from build123d import *

# Parameters (mm, degrees)
F1_DEPTH = 5
F2_W     = 20
F2_H     = 20
F3_DEPTH = 5
F6_W     = 10
F6_H     = 10
F6_R     = 3
F9_DEPTH = 10
F10_R    = 2


with BuildPart() as f1:
    # F0 (on Top) → F1 (new body)
    with BuildSketch(Plane.XY):
        with BuildLine():
            Line((-11.8750007629, -7.425), (-12.575, -7.425))
            Line((-12.575, -7.425), (-13.375, -7.425))
            Line((-13.375, -7.425), (-13.375, -12.575))
            Line((-13.375, -12.575), (-12.575, -12.575))
            Line((-12.575, -12.575), (-11.8750007629, -12.575))
            ThreePointArc((-11.8750007629, -12.575), (-11.6628687671, -12.6628679271), (-11.5750007629, -12.8749998911))
            Line((-11.5750007629, -12.8749998911), (-11.5749999754, -15.0441214738))
            ThreePointArc((-11.5749999754, -15.0441214738), (-11.0934929218, -15.7647472802), (-10.2434566861, -15.5956644799))
            Line((-10.2434566861, -15.5956644799), (-7.9036796566, -13.2558874505))
            ThreePointArc((-7.9036796566, -13.2558874505), (-7.2533614014, -12.2826174011), (-7.0250000001, -11.1345671007))
            Line((-7.0250000001, -11.1345671007), (-7.0250000049, -8.8654328821))
            ThreePointArc((-7.0250000049, -8.8654328821), (-7.2533614085, -7.7173825884), (-7.9036796613, -6.7441125448))
            Line((-7.9036796613, -6.7441125448), (-10.2434566921, -4.404335514))
            ThreePointArc((-10.2434566921, -4.404335514), (-11.0934929289, -4.2352527142), (-11.5749999814, -4.9558785223))
            Line((-11.5749999814, -4.9558785223), (-11.5750007629, -7.1250001081))
            ThreePointArc((-11.5750007629, -7.1250001081), (-11.6628687668, -7.3371320726), (-11.8750007629, -7.425))
        make_face()
    extrude(amount=-F1_DEPTH)



with BuildPart() as f1b:
    # F0 (on Top) → F1, piece 2 (new body)
    with BuildSketch(Plane.XY):
        with BuildLine():
            Line((-0.8, -20), (-0.8, -19.2))
            Line((-0.8, -19.2), (-0.8, -18.5000007629))
            ThreePointArc((-0.8, -18.5000007629), (-0.7121320729, -18.2878687671), (-0.5000001089, -18.2000007629))
            Line((-0.5000001089, -18.2000007629), (1.6691214738, -18.1999999754))
            ThreePointArc((1.6691214738, -18.1999999754), (2.3897472802, -17.7184929218), (2.2206644799, -16.868456686))
            Line((2.2206644799, -16.868456686), (-0.1191125495, -14.5286796566))
            ThreePointArc((-0.1191125495, -14.5286796566), (-1.0923825989, -13.8783614014), (-2.2404328993, -13.6500000001))
            Line((-2.2404328993, -13.6500000001), (-4.5095671179, -13.6500000049))
            ThreePointArc((-4.5095671179, -13.6500000049), (-5.6576174116, -13.8783614085), (-6.6308874552, -14.5286796613))
            Line((-6.6308874552, -14.5286796613), (-8.970664486, -16.8684566921))
            ThreePointArc((-8.970664486, -16.8684566921), (-9.1397472858, -17.7184929288), (-8.4191214777, -18.1999999814))
            Line((-8.4191214777, -18.1999999814), (-6.2499998919, -18.2000007629))
            ThreePointArc((-6.2499998919, -18.2000007629), (-6.0378679274, -18.2878687668), (-5.95, -18.5000007629))
            Line((-5.95, -18.5000007629), (-5.95, -19.2))
            Line((-5.95, -19.2), (-5.95, -20))
            Line((-5.95, -20), (-0.8, -20))
        make_face()
    extrude(amount=-F1_DEPTH)


with BuildPart() as f1c:
    # F0 (on Top) → F1, piece 3 (new body)
    with BuildSketch(Plane.XY):
        with BuildLine():
            Line((3.4934566861, -4.4043355201), (1.1536796566, -6.7441125495))
            ThreePointArc((1.1536796566, -6.7441125495), (0.5033614014, -7.7173825989), (0.2750000001, -8.8654328993))
            Line((0.2750000001, -8.8654328993), (0.2750000049, -11.1345671179))
            ThreePointArc((0.2750000049, -11.1345671179), (0.5033614085, -12.2826174116), (1.1536796613, -13.2558874552))
            Line((1.1536796613, -13.2558874552), (3.4934566921, -15.595664486))
            ThreePointArc((3.4934566921, -15.595664486), (4.3434929289, -15.7647472858), (4.8249999814, -15.0441214777))
            Line((4.8249999814, -15.0441214777), (4.8250007629, -12.8749998919))
            ThreePointArc((4.8250007629, -12.8749998919), (4.9128687668, -12.6628679274), (5.1250007629, -12.575))
            Line((5.1250007629, -12.575), (5.825, -12.575))
            Line((5.825, -12.575), (6.625, -12.575))
            Line((6.625, -12.575), (6.625, -7.425))
            Line((6.625, -7.425), (5.825, -7.425))
            Line((5.825, -7.425), (5.1250007629, -7.425))
            ThreePointArc((5.1250007629, -7.425), (4.9128687671, -7.3371320729), (4.8250007629, -7.1250001089))
            Line((4.8250007629, -7.1250001089), (4.8249999754, -4.9558785262))
            ThreePointArc((4.8249999754, -4.9558785262), (4.3434929218, -4.2352527198), (3.4934566861, -4.4043355201))
        make_face()
    extrude(amount=-F1_DEPTH)


with BuildPart() as f1d:
    # F0 (on Top) → F1, piece 4 (new body)
    with BuildSketch(Plane.XY):
        with BuildLine():
            Line((-0.8, -1.4999992371), (-0.8, -0.8))
            Line((-0.8, -0.8), (-0.8, 0))
            Line((-0.8, 0), (-5.95, 0))
            Line((-5.95, 0), (-5.95, -0.8))
            Line((-5.95, -0.8), (-5.95, -1.4999992371))
            ThreePointArc((-5.95, -1.4999992371), (-6.0378679271, -1.7121312329), (-6.2499998911, -1.7999992371))
            Line((-6.2499998911, -1.7999992371), (-8.4191214738, -1.8000000246))
            ThreePointArc((-8.4191214738, -1.8000000246), (-9.1397472801, -2.2815070782), (-8.9706644799, -3.1315433139))
            Line((-8.9706644799, -3.1315433139), (-6.6308874505, -5.4713203434))
            ThreePointArc((-6.6308874505, -5.4713203434), (-5.6576174011, -6.1216385986), (-4.5095671007, -6.3499999999))
            Line((-4.5095671007, -6.3499999999), (-2.2404328821, -6.3499999951))
            ThreePointArc((-2.2404328821, -6.3499999951), (-1.0923825884, -6.1216385915), (-0.1191125448, -5.4713203387))
            Line((-0.1191125448, -5.4713203387), (2.220664486, -3.1315433079))
            ThreePointArc((2.220664486, -3.1315433079), (2.3897472858, -2.2815070711), (1.6691214777, -1.8000000186))
            Line((1.6691214777, -1.8000000186), (-0.5000001081, -1.7999992371))
            ThreePointArc((-0.5000001081, -1.7999992371), (-0.7121320726, -1.7121312332), (-0.8, -1.4999992371))
        make_face()
    extrude(amount=-F1_DEPTH)


with BuildPart() as f1_1:
    add(f1.part)

    add(f1b.part)  # F3 merges F1b

    add(f1c.part)  # F3 merges F1c

    add(f1d.part)  # F3 merges F1d
    # F2 (on face) → F3 (join)
    with BuildSketch(Plane.XY):
        with Locations((-3.3896967843, -10)):
            Rectangle(F2_W, F2_H)
    extrude(amount=F3_DEPTH)

    # F7: sweep along a path in F5
    with BuildLine(Plane.YZ.offset(-3.3896967843)) as f7_path:
        Line((-25, 0), (-25, 10.8014274722))
        Line((-25, 10.8014274722), (-1.3219409988, 24.4719612104))
    # F6 (on Top) → F7 (sweep)
    with BuildSketch(Plane.XY):
        with Locations((-3.3896967843, -25)):
            Rectangle(F6_W, F6_H)
        with Locations((-3.3896967843, -25)):
            Circle(F6_R, mode=Mode.SUBTRACT)
    sweep(path=f7_path.line, transition=Transition.RIGHT)

    # F8 (on face) → F9 (join)
    with BuildSketch(Plane.YZ.offset(1.6103032157)):
        Polygon((0, 5), (1.1780590012, 20.1418341915), (-20, 7.9146761262), (-20, 5), align=None)
    extrude(amount=-F9_DEPTH)

    # F10
    f10_edges = [f1_1.edges().sort_by_distance(p)[0] for p in [
        (6.610303, 0, 2.5),
        (6.610303, -20, 2.5),
        (-13.389697, 0, 2.5),
        (-13.389697, -20, 2.5),
        (-8.389697, -30, 6.844089),
        (1.610303, -30, 6.844089),
        (-8.389697, -16.91097, 21.245134),
        (1.610303, -16.91097, 21.245134),
        (-3.389697, -30, 13.688179),
        (-8.389697, -20, 2.5),
        (1.610303, -20, 2.5),
        (1.610303, -10, 5),
        (-8.389697, -10, 5),
        (-3.389697, 1.178059, 20.141834),
    ]]
    fillet(f10_edges, radius=F10_R)


solid = f1_1.part
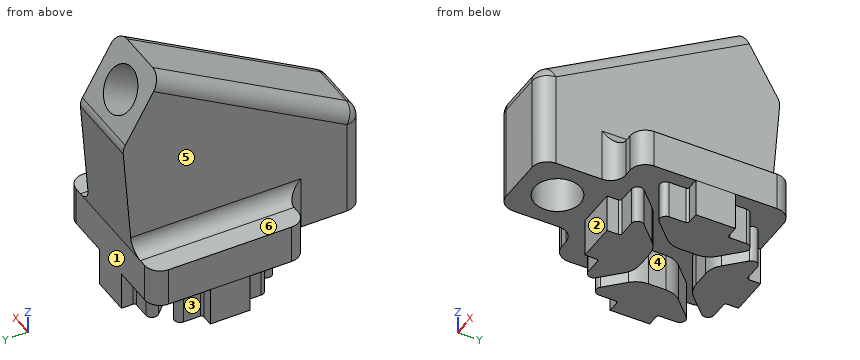
Build history of the part. All positions in model axes, mm. Face numbers are marked on the shaded views. A direction names the side the tool comes from. Give positions to 0.01 mm unless a question says otherwise; leave off trailing zeros. Write item = value, one per line. Start each with the question number.
1) Pull direction X, two halves, no side cores. Call the marked faces 4, 5 and 6: +X half, -X half, draft (parallel to the pull), parting line (faces both ways), or undercut.
2) Tool access for the marked faces 1, 2 and 3: list every direction of +Z, -Z, +X, -X, +Y, -Y with a clear straight run to the whole face (end or side of a thin tool).
3) Probe probe 1 along X at (y, z) = (-25, 5); probe 2 along Y at (x, z) = (-1.25, 14); probe 3 along X at (y, z) = (-22.5, 13.5). List the from-to ranges inside material, lowest first. Write a range as from..to.
4) Band-saw the part on A-A on z = -2. Count the separate pieces of the cut face and the enclosed holes in it, plus the area to 3 significant figures.
5) Drop flat-ended pins along their axis: pin 1 Ø10 at (y, z) = (-6, 17.5) entering from -X; pin 2 Ø5 at (x, y) = (-3.39, -25) entering from +Z; pin 3 Ø0.9 at (x, y) = (4.5, -5) entering from +Z. Give the stop position or say it passes through.
Final values:
q1.face_4 = undercut
q1.face_5 = -X half
q1.face_6 = draft
q2.face_1 = -Z, +X, -X, +Y
q2.face_2 = -Z, +X, -X, -Y
q2.face_3 = -Z, -X, +Y
q3.probe_1 = -8.39..-6.39, -0.39..1.61
q3.probe_2 = -29.36..-23.67, -15.25..0.7
q3.probe_3 = -8.39..-6.19, -0.59..1.61
q4.separate_pieces = 4
q4.enclosed_holes = 0
q4.area = 199 mm²
q5.pin_1 = -8.39
q5.pin_2 = 18.02
q5.pin_3 = 5
